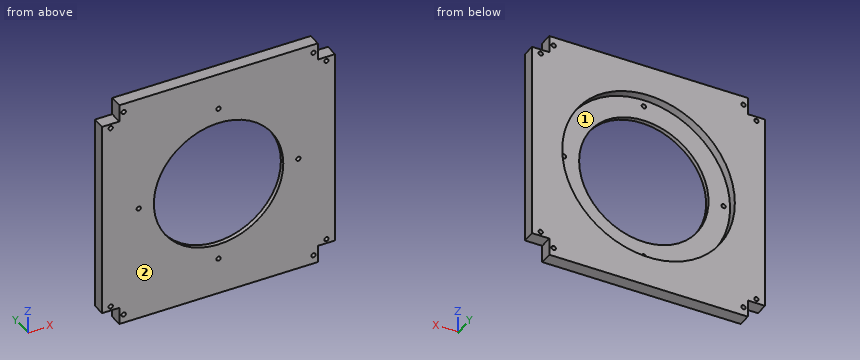
```python
from build123d import *

# Parameters (mm, degrees)
SKETCH1_W           = 270
SKETCH1_H           = 270
BOSS_EXTRUDE1_DEPTH = 15
SKETCH8_W           = 20
SKETCH8_H           = 20
CUT_EXTRUDE1_DEPTH  = 16
SKETCH9_R           = 2.5
CUT_EXTRUDE2_DEPTH  = 16
SKETCH10_R          = 100
CUT_EXTRUDE3_DEPTH  = 10
SKETCH12_R          = 75
SKETCH12_R_2        = 2.5
CUT_EXTRUDE4_DEPTH  = 6


with BuildPart() as part:
    # Sketch1 → Boss-Extrude1 (new body)
    with BuildSketch(Plane(origin=(0, 0, 0), x_dir=(1, 0, 0), z_dir=(0, 1, 0))):
        with Locations((135, 135)):
            Rectangle(SKETCH1_W, SKETCH1_H)
    extrude(amount=BOSS_EXTRUDE1_DEPTH)

    # Sketch8 → Cut-Extrude1 (cut, through all)
    with BuildSketch(Plane(origin=(0, 15, 0), x_dir=(1, 0, 0), z_dir=(0, 1, 0))):
        with Locations((10, 260)):
            Rectangle(SKETCH8_W, SKETCH8_H)
        with Locations((260, 260)):
            Rectangle(SKETCH8_W, SKETCH8_H)
        with Locations((260, 10)):
            Rectangle(SKETCH8_W, SKETCH8_H)
        with Locations((10, 10)):
            Rectangle(SKETCH8_W, SKETCH8_H)
    extrude(amount=-CUT_EXTRUDE1_DEPTH, mode=Mode.SUBTRACT)

    # Sketch9 → Cut-Extrude2 (cut, through all)
    with BuildSketch(Plane(origin=(0, 15, 0), x_dir=(1, 0, 0), z_dir=(0, 1, 0))):
        with Locations((10, 245)):
            Circle(SKETCH9_R)
        with Locations((10, 25)):
            Circle(SKETCH9_R)
        with Locations((25, 10)):
            Circle(SKETCH9_R)
        with Locations((245, 10)):
            Circle(SKETCH9_R)
        with Locations((260, 25)):
            Circle(SKETCH9_R)
        with Locations((260, 245)):
            Circle(SKETCH9_R)
        with Locations((245, 260)):
            Circle(SKETCH9_R)
        with Locations((25, 260)):
            Circle(SKETCH9_R)
    extrude(amount=-CUT_EXTRUDE2_DEPTH, mode=Mode.SUBTRACT)

    # Sketch10 → Cut-Extrude3 (cut)
    with BuildSketch(Plane(origin=(0, 15, 0), x_dir=(1, 0, 0), z_dir=(0, 1, 0))):
        with Locations((135, 135)):
            Circle(SKETCH10_R)
    extrude(amount=-CUT_EXTRUDE3_DEPTH, mode=Mode.SUBTRACT)

    # Sketch12 → Cut-Extrude4 (cut, through all)
    with BuildSketch(Plane(origin=(0, 5, 0), x_dir=(1, 0, 0), z_dir=(0, 1, 0))):
        with Locations((135, 135)):
            Circle(SKETCH12_R)
        with Locations((135, 227.5)):
            Circle(SKETCH12_R_2)
        with Locations((227.5, 135)):
            Circle(SKETCH12_R_2)
        with Locations((135, 42.5)):
            Circle(SKETCH12_R_2)
        with Locations((42.5, 135)):
            Circle(SKETCH12_R_2)
    extrude(amount=-CUT_EXTRUDE4_DEPTH, mode=Mode.SUBTRACT)


solid = part.part
```
Build history of the part. All positions in model axes, mm. Face numbers are marked on the shaded views. Give positions to 0.01 mm unless a question says otherwise; leave off trailing zeros. Loops run counter-clockwise (first coordinate to the right, second up) from the corner with the lowest first, then second, coordinate; pieces in that order, holes last.
1) Probe line 1 along Z through (x, y) = (260, 7); line 2 along Z through (x, y) = (25, 9.75); line 3 along X through (y, z) = (7.5, -25). List the from-to ranges inside material, lowest first.
Values follow:
line 1: z = -250 to -247.5, -242.5 to -27.5, -22.5 to -20
line 2: z = -270 to -262.5, -257.5 to -12.5, -7.5 to 0
line 3: x = 0 to 7.5, 12.5 to 257.5, 262.5 to 270
2) Drop flat-ended pins along their axis: P1, Ø7.5, axis at x = 257.5, y = 8.5, coming from the +Z side; P2, Ø4.5, axis at x = 15, y = 10.5, coming from the -Z side; P3, Ø6, axis at x = 135, z = -227.5, coming from the +Y side. Give the stop position or say it passes through.
Values follow:
P1: stops at z = -20
P2: stops at z = -250
P3: stops at y = 5
3) Two-plate mould, pull along Z, no slides. Class the marked faces 1 and 2: released by +Z, released by -Z, zero draft, split by the parting line, or undercut.
Values follow:
face 1: undercut
face 2: zero draft
4) Band-saw the part on B-B on z = -141. List the corners of the cut face in (x, y).
Values follow:
outline: (0, 0) - (60.24, 0) - (60.24, 5) - (35.18, 5) - (35.18, 15) - (0, 15) - close; (209.76, 0) - (270, 0) - (270, 15) - (234.82, 15) - (234.82, 5) - (209.76, 5) - close
5) Band-saw the part on A-A on y = 12. State how many separate pieces and enclosed holes the cut face has, then the cut area to 3 significant figures.
Values follow:
separate pieces: 1
enclosed holes: 9
area: 39,700 mm2
6) Band-saw the part on C-C on x = 118. List the corners of the cut face in (y, z), then the cut area to 3 significant figures.
Values follow:
outline: (0, -270) - (15, -270) - (15, -233.54) - (5, -233.54) - (5, -208.05) - (0, -208.05) - close; (0, -61.95) - (5, -61.95) - (5, -36.46) - (15, -36.46) - (15, 0) - (0, 0) - close
area: 1,350 mm2
